```python
from build123d import *

# Parameters (mm, degrees)
F0_R     = 3.375
F0_R_2   = 1.95
F1_DEPTH = 3
F0_R_3   = 3.25
F2_DEPTH = 1.7
F3_DEPTH = 3
F4_R     = 3.375
F5_DEPTH = 2.25
F6_R     = 4.5310889132
F7_DEPTH = 3.75
F8_R     = 0.75


# Not quite as in the source:
# - a feature names something its author has since deleted; it is built from what else it names


with BuildPart() as f1:
    # F0 (on Top) → F1 (new body)
    with BuildSketch(Plane.XY):
        with BuildLine():
            ThreePointArc((16.6, 0), (0, 16.6), (-16.6, 0))
            ThreePointArc((-16.6, 0), (0, -16.6), (16.6, 0))
        make_face()
        with BuildLine():
            ThreePointArc((14.9348958333, 1.3960252317), (14.9837151184, 0.698771243), (15, 0))
            ThreePointArc((15, 0), (14.9837151184, -0.698771243), (14.9348958333, -1.3960252317))
            ThreePointArc((14.9348958333, -1.3960252317), (10.6066017178, -10.6066017178), (1.3960252317, -14.9348958333))
            ThreePointArc((1.3960252317, -14.9348958333), (0, -15), (-1.3960252317, -14.9348958333))
            ThreePointArc((-1.3960252317, -14.9348958333), (-10.6066017178, -10.6066017178), (-14.9348958333, -1.3960252317))
            ThreePointArc((-14.9348958333, -1.3960252317), (-14.9837151184, -0.698771243), (-15, 0))
            ThreePointArc((-15, 0), (-14.9837151184, 0.698771243), (-14.9348958333, 1.3960252317))
            ThreePointArc((-14.9348958333, 1.3960252317), (-10.6066017178, 10.6066017178), (-1.3960252317, 14.9348958333))
            ThreePointArc((-1.3960252317, 14.9348958333), (0, 15), (1.3960252317, 14.9348958333))
            ThreePointArc((1.3960252317, 14.9348958333), (10.6066017178, 10.6066017178), (14.9348958333, 1.3960252317))
        make_face(mode=Mode.SUBTRACT)
        with BuildLine():
            ThreePointArc((1.25, -4.3229041164), (3.1819805153, -3.1819805153), (4.3229041164, -1.25))
            ThreePointArc((4.3229041164, -1.25), (4.4555060613, -0.6312414261), (4.5, 0))
            ThreePointArc((4.5, 0), (4.4555060613, 0.6312414261), (4.3229041164, 1.25))
            ThreePointArc((4.3229041164, 1.25), (3.1819805153, 3.1819805153), (1.25, 4.3229041164))
            ThreePointArc((1.25, 4.3229041164), (0, 4.5), (-1.25, 4.3229041164))
            ThreePointArc((-1.25, 4.3229041164), (-3.1819805153, 3.1819805153), (-4.3229041164, 1.25))
            ThreePointArc((-4.3229041164, 1.25), (-4.5, 0), (-4.3229041164, -1.25))
            ThreePointArc((-4.3229041164, -1.25), (-3.1819805153, -3.1819805153), (-1.25, -4.3229041164))
            ThreePointArc((-1.25, -4.3229041164), (0, -4.5), (1.25, -4.3229041164))
        make_face()
        Circle(F0_R, mode=Mode.SUBTRACT)
        Circle(F0_R)
        Polygon((-2.25, 0), (-1.125, 1.9485571585), (1.125, 1.9485571585), (2.25, 0), (1.125, -1.9485571585), (-1.125, -1.9485571585), align=None, mode=Mode.SUBTRACT)
        with BuildLine():
            ThreePointArc((14.9348958333, -1.3960252317), (14.9837151184, -0.698771243), (15, 0))
            ThreePointArc((15, 0), (14.9837151184, 0.698771243), (14.9348958333, 1.3960252317))
            ThreePointArc((14.9348958333, 1.3960252317), (11.9200595209, 3.2490167004), (9, 1.25))
            ThreePointArc((9, 1.25), (8.75, 0), (9, -1.25))
            ThreePointArc((9, -1.25), (11.9200595209, -3.2490167004), (14.9348958333, -1.3960252317))
        make_face()
        with Locations((12, 0)):
            Circle(F0_R_2, mode=Mode.SUBTRACT)
        with BuildLine():
            ThreePointArc((1.25, 9), (3.2490167004, 11.9200595209), (1.3960252317, 14.9348958333))
            ThreePointArc((1.3960252317, 14.9348958333), (0, 15), (-1.3960252317, 14.9348958333))
            ThreePointArc((-1.3960252317, 14.9348958333), (-3.2490167004, 11.9200595209), (-1.25, 9))
            ThreePointArc((-1.25, 9), (0, 8.75), (1.25, 9))
        make_face()
        with Locations((0, 12)):
            Circle(F0_R_2, mode=Mode.SUBTRACT)
        with BuildLine():
            ThreePointArc((-1.3960252317, -14.9348958333), (0, -15), (1.3960252317, -14.9348958333))
            ThreePointArc((1.3960252317, -14.9348958333), (3.2490167004, -11.9200595209), (1.25, -9))
            ThreePointArc((1.25, -9), (0, -8.75), (-1.25, -9))
            ThreePointArc((-1.25, -9), (-3.2490167004, -11.9200595209), (-1.3960252317, -14.9348958333))
        make_face()
        with Locations((0, -12)):
            Circle(F0_R_2, mode=Mode.SUBTRACT)
        with BuildLine():
            ThreePointArc((-9, 1.25), (-11.9200595209, 3.2490167004), (-14.9348958333, 1.3960252317))
            ThreePointArc((-14.9348958333, 1.3960252317), (-14.9837151184, 0.698771243), (-15, 0))
            ThreePointArc((-15, 0), (-14.9837151184, -0.698771243), (-14.9348958333, -1.3960252317))
            ThreePointArc((-14.9348958333, -1.3960252317), (-11.9200595209, -3.2490167004), (-9, -1.25))
            ThreePointArc((-9, -1.25), (-8.75, 0), (-9, 1.25))
        make_face()
        with Locations((-12, 0)):
            Circle(F0_R_2, mode=Mode.SUBTRACT)
        with BuildLine():
            ThreePointArc((9, -1.25), (8.75, 0), (9, 1.25))
            Line((9, 1.25), (6, 1.25))
            Line((6, 1.25), (4.3229041164, 1.25))
            ThreePointArc((4.3229041164, 1.25), (4.4555060613, 0.6312414261), (4.5, 0))
            ThreePointArc((4.5, 0), (4.4555060613, -0.6312414261), (4.3229041164, -1.25))
            Line((4.3229041164, -1.25), (9, -1.25))
        make_face()
        with BuildLine():
            Line((1.25, 4.3229041164), (1.25, 9))
            ThreePointArc((1.25, 9), (0, 8.75), (-1.25, 9))
            Line((-1.25, 9), (-1.25, 6))
            Line((-1.25, 6), (-1.25, 4.3229041164))
            ThreePointArc((-1.25, 4.3229041164), (0, 4.5), (1.25, 4.3229041164))
        make_face()
        with BuildLine():
            ThreePointArc((-1.25, -9), (0, -8.75), (1.25, -9))
            Line((1.25, -9), (1.25, -6))
            Line((1.25, -6), (1.25, -4.3229041164))
            ThreePointArc((1.25, -4.3229041164), (0, -4.5), (-1.25, -4.3229041164))
            Line((-1.25, -4.3229041164), (-1.25, -9))
        make_face()
        with BuildLine():
            Line((-4.3229041164, 1.25), (-9, 1.25))
            ThreePointArc((-9, 1.25), (-8.75, 0), (-9, -1.25))
            Line((-9, -1.25), (-6, -1.25))
            Line((-6, -1.25), (-4.3229041164, -1.25))
            ThreePointArc((-4.3229041164, -1.25), (-4.5, 0), (-4.3229041164, 1.25))
        make_face()
    extrude(amount=F1_DEPTH)



with BuildPart() as f1b:
    # F0 (on Top) → F1, piece 2 (new body)
    with BuildSketch(Plane.XY):
        with Locations((6.8942911166, 6.8942911166)):
            Circle(F0_R_3)
        with Locations((6.8942911166, 6.8942911166)):
            Circle(F0_R_2, mode=Mode.SUBTRACT)
    extrude(amount=F1_DEPTH)


with BuildPart() as f1c:
    # F0 (on Top) → F1, piece 3 (new body)
    with BuildSketch(Plane.XY):
        with Locations((-6.8942911166, 6.8942911166)):
            Circle(F0_R_3)
        with Locations((-6.8942911166, 6.8942911166)):
            Circle(F0_R_2, mode=Mode.SUBTRACT)
    extrude(amount=F1_DEPTH)


with BuildPart() as f1d:
    # F0 (on Top) → F1, piece 4 (new body)
    with BuildSketch(Plane.XY):
        with Locations((-6.8942911166, -6.8942911166)):
            Circle(F0_R_3)
        with Locations((-6.8942911166, -6.8942911166)):
            Circle(F0_R_2, mode=Mode.SUBTRACT)
    extrude(amount=F1_DEPTH)


with BuildPart() as f1e:
    # F0 (on Top) → F1, piece 5 (new body)
    with BuildSketch(Plane.XY):
        with Locations((6.8942911166, -6.8942911166)):
            Circle(F0_R_3)
        with Locations((6.8942911166, -6.8942911166)):
            Circle(F0_R_2, mode=Mode.SUBTRACT)
    extrude(amount=F1_DEPTH)


with BuildPart() as f1_1:
    add(f1.part)

    add(f1b.part)  # F2 merges F1b

    add(f1c.part)  # F2 merges F1c

    add(f1d.part)  # F2 merges F1d

    add(f1e.part)  # F2 merges F1e
    # F0 (on Top) → F2 (join)
    with BuildSketch(Plane.XY):
        with BuildLine():
            ThreePointArc((-1.25, 9), (-3.2490167004, 11.9200595209), (-1.3960252317, 14.9348958333))
            ThreePointArc((-1.3960252317, 14.9348958333), (-10.6066017178, 10.6066017178), (-14.9348958333, 1.3960252317))
            ThreePointArc((-14.9348958333, 1.3960252317), (-11.9200595209, 3.2490167004), (-9, 1.25))
            Line((-9, 1.25), (-4.3229041164, 1.25))
            ThreePointArc((-4.3229041164, 1.25), (-3.1819805153, 3.1819805153), (-1.25, 4.3229041164))
            Line((-1.25, 4.3229041164), (-1.25, 6))
            Line((-1.25, 6), (-1.25, 9))
        make_face()
        with Locations((-6.8942911166, 6.8942911166)):
            Circle(F0_R_3, mode=Mode.SUBTRACT)
        with BuildLine():
            ThreePointArc((9, 1.25), (11.9200595209, 3.2490167004), (14.9348958333, 1.3960252317))
            ThreePointArc((14.9348958333, 1.3960252317), (10.6066017178, 10.6066017178), (1.3960252317, 14.9348958333))
            ThreePointArc((1.3960252317, 14.9348958333), (3.2490167004, 11.9200595209), (1.25, 9))
            Line((1.25, 9), (1.25, 4.3229041164))
            ThreePointArc((1.25, 4.3229041164), (3.1819805153, 3.1819805153), (4.3229041164, 1.25))
            Line((4.3229041164, 1.25), (6, 1.25))
            Line((6, 1.25), (9, 1.25))
        make_face()
        with Locations((6.8942911166, 6.8942911166)):
            Circle(F0_R_3, mode=Mode.SUBTRACT)
        with BuildLine():
            ThreePointArc((1.3960252317, -14.9348958333), (10.6066017178, -10.6066017178), (14.9348958333, -1.3960252317))
            ThreePointArc((14.9348958333, -1.3960252317), (11.9200595209, -3.2490167004), (9, -1.25))
            Line((9, -1.25), (4.3229041164, -1.25))
            ThreePointArc((4.3229041164, -1.25), (3.1819805153, -3.1819805153), (1.25, -4.3229041164))
            Line((1.25, -4.3229041164), (1.25, -6))
            Line((1.25, -6), (1.25, -9))
            ThreePointArc((1.25, -9), (3.2490167004, -11.9200595209), (1.3960252317, -14.9348958333))
        make_face()
        with Locations((6.8942911166, -6.8942911166)):
            Circle(F0_R_3, mode=Mode.SUBTRACT)
        with BuildLine():
            ThreePointArc((-14.9348958333, -1.3960252317), (-10.6066017178, -10.6066017178), (-1.3960252317, -14.9348958333))
            ThreePointArc((-1.3960252317, -14.9348958333), (-3.2490167004, -11.9200595209), (-1.25, -9))
            Line((-1.25, -9), (-1.25, -4.3229041164))
            ThreePointArc((-1.25, -4.3229041164), (-3.1819805153, -3.1819805153), (-4.3229041164, -1.25))
            Line((-4.3229041164, -1.25), (-6, -1.25))
            Line((-6, -1.25), (-9, -1.25))
            ThreePointArc((-9, -1.25), (-11.9200595209, -3.2490167004), (-14.9348958333, -1.3960252317))
        make_face()
        with Locations((-6.8942911166, -6.8942911166)):
            Circle(F0_R_3, mode=Mode.SUBTRACT)
        Circle(F0_R)
        Polygon((-2.25, 0), (-1.125, 1.9485571585), (1.125, 1.9485571585), (2.25, 0), (1.125, -1.9485571585), (-1.125, -1.9485571585), align=None, mode=Mode.SUBTRACT)
    extrude(amount=F2_DEPTH)

    # F0 (on Top) → F3 (join)
    with BuildSketch(Plane.XY):
        with BuildLine():
            ThreePointArc((16.6, 0), (0, 16.6), (-16.6, 0))
            ThreePointArc((-16.6, 0), (0, -16.6), (16.6, 0))
        make_face()
        with BuildLine():
            ThreePointArc((14.9348958333, 1.3960252317), (14.9837151184, 0.698771243), (15, 0))
            ThreePointArc((15, 0), (14.9837151184, -0.698771243), (14.9348958333, -1.3960252317))
            ThreePointArc((14.9348958333, -1.3960252317), (10.6066017178, -10.6066017178), (1.3960252317, -14.9348958333))
            ThreePointArc((1.3960252317, -14.9348958333), (0, -15), (-1.3960252317, -14.9348958333))
            ThreePointArc((-1.3960252317, -14.9348958333), (-10.6066017178, -10.6066017178), (-14.9348958333, -1.3960252317))
            ThreePointArc((-14.9348958333, -1.3960252317), (-14.9837151184, -0.698771243), (-15, 0))
            ThreePointArc((-15, 0), (-14.9837151184, 0.698771243), (-14.9348958333, 1.3960252317))
            ThreePointArc((-14.9348958333, 1.3960252317), (-10.6066017178, 10.6066017178), (-1.3960252317, 14.9348958333))
            ThreePointArc((-1.3960252317, 14.9348958333), (0, 15), (1.3960252317, 14.9348958333))
            ThreePointArc((1.3960252317, 14.9348958333), (10.6066017178, 10.6066017178), (14.9348958333, 1.3960252317))
        make_face(mode=Mode.SUBTRACT)
    extrude(amount=F3_DEPTH)

    # F4 (on face) → F5 (cut)
    with BuildSketch(Plane.XY.offset(3)):
        Circle(F4_R)
        Polygon((-1.125, 1.9485571585), (1.125, 1.9485571585), (2.25, 0), (1.125, -1.9485571585), (-1.125, -1.9485571585), (-2.25, 0), align=None, mode=Mode.SUBTRACT)
    extrude(amount=-F5_DEPTH, mode=Mode.SUBTRACT)

    # F6 (on face) → F7 (join)
    with BuildSketch(Plane(origin=(0, 0, 0), x_dir=(1, 0, 0), z_dir=(0, 0, -1))):
        Circle(F6_R)
        Polygon((-3.5, 0), (-1.75, 3.0310889132), (1.75, 3.0310889132), (3.5, 0), (1.75, -3.0310889132), (-1.75, -3.0310889132), align=None, mode=Mode.SUBTRACT)
    extrude(amount=F7_DEPTH)

    # F8
    f8_edges = [f1_1.edges().sort_by_distance(p)[0] for p in [
        (-4.531089, 0, -3.75),
    ]]
    fillet(f8_edges, radius=F8_R)


solid = f1_1.part
```
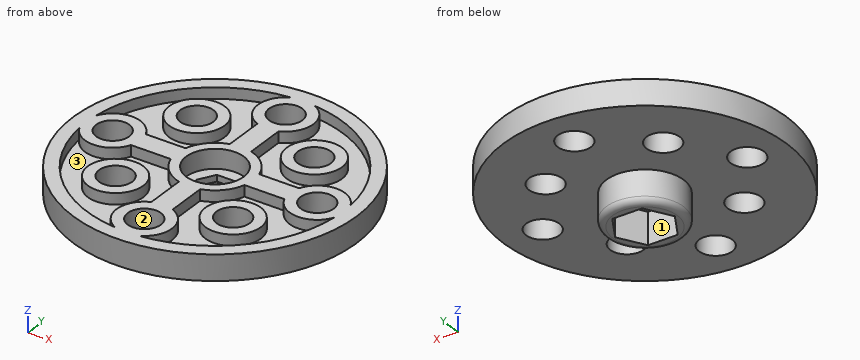
Check sheet for the modelled part. Datum: model origin and axes. Units: mm. Face numbers are marked on the shaded views. A direction names the side the tool comes from. Coordinates: 2 decimals unless noted, no trailing zeros. Loops run counter-clockwise (first coordinate to the right, second up) from the corner with the lowest first, then second, coordinate; pieces in that order, holes last.
1) Sectioned sample at A-A (x = 0). Count the separate pieces of the cut face and the enclosed holes in it, and give its area (3 significant figures).
2) Gauge pin test, flat ends, axial feed: pin 1 (2 mm diameter, centred on x = 6.5, y = 8.5, fed in from -Z); pin 2 (1 mm diameter, centred on y = -5.5, z = 2.5, fed in from -X); pin 3 (1.4 mm diameter, centred on x = -6.5, z = 2.5, fed in from +Y). Record the tip position at first contact, or that the pin passes through.
3) Sectioned sample at B-B (z = -1.75). Record the boundary of the cut face in (x, y), and give its area (3 significant figures).
4) Sectioned sample at C-C (y = 12). Record the boundary of the cut face in (x, z).
5) Access from +Z, -Z, +X, -X, +Y, -Y to the whole of each face (thin tool, end or side, straight path). Record for the marked faces 1, 2 and 3.
6) Sectioned sample at D-D (y = 7.5). Record the boundary of the cut face in (x, z).
7) Material ranges on probe 1 along Y at (x, z) = (0, 1.45) (3 decimals); probe 2 along Y at (x, z) = (7, 0.5); probe 3 along Z at (x, y) = (13.5, -9), recorded low to high.
Check sheet entries:
1. separate pieces: 4
1. enclosed holes: 0
1. area: 69.1 mm2
2. pin 1: stops at z = 0
2. pin 2: stops at x = -15.83
2. pin 3: stops at y = 15.55
3. outline: circle Ø9.06 at (0, 0); hole (-3.5, 0) - (-1.75, -3.03) - (1.75, -3.03) - (3.5, 0) - (1.75, 3.03) - (-1.75, 3.03) - close
3. area: 32.7 mm2
4. outline: (-11.47, 0) - (-1.95, 0) - (-1.95, 3) - (-3.25, 3) - (-3.25, 1.7) - (-9, 1.7) - (-9, 3) - (-11.47, 3) - close; (1.95, 0) - (11.47, 0) - (11.47, 3) - (9, 3) - (9, 1.7) - (3.25, 1.7) - (3.25, 3) - (1.95, 3) - close
5. face 1: -Z
5. face 2: +Z, -Z
5. face 3: +Z
6. outline: (-14.81, 0) - (-8.75, 0) - (-8.75, 3) - (-10.09, 3) - (-10.09, 1.7) - (-12.99, 1.7) - (-12.99, 3) - (-14.81, 3) - close; (-5.04, 0) - (5.04, 0) - (5.04, 3) - (3.7, 3) - (3.7, 1.7) - (1.25, 1.7) - (1.25, 3) - (-1.25, 3) - (-1.25, 1.7) - (-3.7, 1.7) - (-3.7, 3) - (-5.04, 3) - close; (8.75, 0) - (14.81, 0) - (14.81, 3) - (12.99, 3) - (12.99, 1.7) - (10.09, 1.7) - (10.09, 3) - (8.75, 3) - close
7. probe 1: y = -16.6 to -13.95, -10.05 to -3.375, 3.375 to 10.05, 13.95 to 16.6
7. probe 2: y = -15.05 to -8.84, -4.95 to 4.95, 8.84 to 15.05
7. probe 3: z = 0 to 3
